from build123d import *

# Parameters (mm, degrees)
F0_W           = 85
F0_H           = 85
F0_W_2         = 80
F0_H_2         = 80
F1_DEPTH       = 5
F0_R           = 3.25
F2_DEPTH       = 2.5
F3_D           = 3
F3_CSINK_D     = 5.75
F3_CSINK_ANGLE = 90


with BuildPart() as f1:
    # F0 (on Top) → F1 (new body)
    with BuildSketch(Plane.XY):
        Rectangle(F0_W, F0_H)
        Rectangle(F0_W_2, F0_H_2, mode=Mode.SUBTRACT)
    extrude(amount=-F1_DEPTH)

    # F0 (on Top) → F2 (join)
    with BuildSketch(Plane.XY):
        Rectangle(F0_W_2, F0_H_2)
        with Locations((-35, -35)):
            Circle(F0_R, mode=Mode.SUBTRACT)
        with Locations((-25, -35)):
            Circle(F0_R, mode=Mode.SUBTRACT)
        with Locations((-35, -25)):
            Circle(F0_R, mode=Mode.SUBTRACT)
        with Locations((-15, -35)):
            Circle(F0_R, mode=Mode.SUBTRACT)
        with Locations((-5, -35)):
            Circle(F0_R, mode=Mode.SUBTRACT)
        with Locations((-15, -25)):
            Circle(F0_R, mode=Mode.SUBTRACT)
        with Locations((-5, -25)):
            Circle(F0_R, mode=Mode.SUBTRACT)
        with Locations((-35, -15)):
            Circle(F0_R, mode=Mode.SUBTRACT)
        with Locations((-25, -15)):
            Circle(F0_R, mode=Mode.SUBTRACT)
        with Locations((-35, -5)):
            Circle(F0_R, mode=Mode.SUBTRACT)
        with Locations((-25, -5)):
            Circle(F0_R, mode=Mode.SUBTRACT)
        with Locations((-15, -15)):
            Circle(F0_R, mode=Mode.SUBTRACT)
        with Locations((-5, -15)):
            Circle(F0_R, mode=Mode.SUBTRACT)
        with Locations((-15, -5)):
            Circle(F0_R, mode=Mode.SUBTRACT)
        with Locations((-5, -5)):
            Circle(F0_R, mode=Mode.SUBTRACT)
        with Locations((5, -35)):
            Circle(F0_R, mode=Mode.SUBTRACT)
        with Locations((15, -35)):
            Circle(F0_R, mode=Mode.SUBTRACT)
        with Locations((5, -25)):
            Circle(F0_R, mode=Mode.SUBTRACT)
        with Locations((15, -25)):
            Circle(F0_R, mode=Mode.SUBTRACT)
        with Locations((25, -35)):
            Circle(F0_R, mode=Mode.SUBTRACT)
        with Locations((35, -35)):
            Circle(F0_R, mode=Mode.SUBTRACT)
        with Locations((35, -25)):
            Circle(F0_R, mode=Mode.SUBTRACT)
        with Locations((5, -15)):
            Circle(F0_R, mode=Mode.SUBTRACT)
        with Locations((15, -15)):
            Circle(F0_R, mode=Mode.SUBTRACT)
        with Locations((5, -5)):
            Circle(F0_R, mode=Mode.SUBTRACT)
        with Locations((15, -5)):
            Circle(F0_R, mode=Mode.SUBTRACT)
        with Locations((25, -15)):
            Circle(F0_R, mode=Mode.SUBTRACT)
        with Locations((35, -15)):
            Circle(F0_R, mode=Mode.SUBTRACT)
        with Locations((25, -5)):
            Circle(F0_R, mode=Mode.SUBTRACT)
        with Locations((35, -5)):
            Circle(F0_R, mode=Mode.SUBTRACT)
        with Locations((-35, 5)):
            Circle(F0_R, mode=Mode.SUBTRACT)
        with Locations((-25, 5)):
            Circle(F0_R, mode=Mode.SUBTRACT)
        with Locations((-35, 15)):
            Circle(F0_R, mode=Mode.SUBTRACT)
        with Locations((-25, 15)):
            Circle(F0_R, mode=Mode.SUBTRACT)
        with Locations((-15, 5)):
            Circle(F0_R, mode=Mode.SUBTRACT)
        with Locations((-5, 5)):
            Circle(F0_R, mode=Mode.SUBTRACT)
        with Locations((-15, 15)):
            Circle(F0_R, mode=Mode.SUBTRACT)
        with Locations((-5, 15)):
            Circle(F0_R, mode=Mode.SUBTRACT)
        with Locations((-35, 25)):
            Circle(F0_R, mode=Mode.SUBTRACT)
        with Locations((-35, 35)):
            Circle(F0_R, mode=Mode.SUBTRACT)
        with Locations((-25, 35)):
            Circle(F0_R, mode=Mode.SUBTRACT)
        with Locations((-15, 25)):
            Circle(F0_R, mode=Mode.SUBTRACT)
        with Locations((-5, 25)):
            Circle(F0_R, mode=Mode.SUBTRACT)
        with Locations((-15, 35)):
            Circle(F0_R, mode=Mode.SUBTRACT)
        with Locations((-5, 35)):
            Circle(F0_R, mode=Mode.SUBTRACT)
        with Locations((5, 5)):
            Circle(F0_R, mode=Mode.SUBTRACT)
        with Locations((15, 5)):
            Circle(F0_R, mode=Mode.SUBTRACT)
        with Locations((5, 15)):
            Circle(F0_R, mode=Mode.SUBTRACT)
        with Locations((15, 15)):
            Circle(F0_R, mode=Mode.SUBTRACT)
        with Locations((25, 5)):
            Circle(F0_R, mode=Mode.SUBTRACT)
        with Locations((35, 5)):
            Circle(F0_R, mode=Mode.SUBTRACT)
        with Locations((25, 15)):
            Circle(F0_R, mode=Mode.SUBTRACT)
        with Locations((35, 15)):
            Circle(F0_R, mode=Mode.SUBTRACT)
        with Locations((5, 25)):
            Circle(F0_R, mode=Mode.SUBTRACT)
        with Locations((15, 25)):
            Circle(F0_R, mode=Mode.SUBTRACT)
        with Locations((5, 35)):
            Circle(F0_R, mode=Mode.SUBTRACT)
        with Locations((15, 35)):
            Circle(F0_R, mode=Mode.SUBTRACT)
        with Locations((35, 25)):
            Circle(F0_R, mode=Mode.SUBTRACT)
        with Locations((25, 35)):
            Circle(F0_R, mode=Mode.SUBTRACT)
        with Locations((35, 35)):
            Circle(F0_R, mode=Mode.SUBTRACT)
    extrude(amount=-F2_DEPTH)

    # F3 (through all)
    with Locations(Plane.XY):
        with Locations((-25, 25), (25, 25), (25, -25), (-25, -25)):
            CounterSinkHole(F3_D / 2, F3_CSINK_D / 2, counter_sink_angle=F3_CSINK_ANGLE)


solid = f1.part
Work out the finished part from the listing and answer in its coordinate system (mm). A direction names the side the tool comes from. Coordinates: 2 decimals unless noted, no trailing zeros. Order: outer loops, then holes, each group sorted by start corner. A loop starts at its lowest first (then second) coordinate and runs counter-clockwise, first axis right, second up. Notation, with made-up numbers: (31, 3) - (37, 3) arc R23 cw to (37, 29) - close; hole circle Ø6 at (55, 32.5). An arc over 180 degrees is marked (long way). Put each result on its own line as item: value. Start each with the question number.
1) Find the intervals of material crossed by line 1 (X direction, y = -16, z = -4.4); line 2 (Z direction, x = -16.5, y = 11), in increasing order. Write a range as from..to.
2) Find section A-A (y = 0). Give the vertices of the cut face in (x, z), plus the area to 3 significant figures.
3) For faces 3 (the cylindrical face through (-33.5, -37.883, -1.232)), 4 (the flat face through (-40, -1, -4)), determine the directions among +Z, -Z, +X, -X, +Y, -Y from which every point of the face is accessible in a straight line to the end or side of a thin tool.
4) For a pull along Y with two mould halves and no side action, classify faces 1 (the flat face through (-1, 1, 0)), 2 (the cylindrical face through (14.295, -38.173, -1.232)) as released by +Y, released by -Y, zero draft, split by the parting line, or undercut.
5) Flat-ended cylindrical pins translate along their axes: pin 1 (7.5 mm diameter, centred on x = -5, y = -35, fed in from -Z); pin 2 (4 mm diameter, centred on x = -35, y = -5, fed in from -Z). Find the tip coordinate at first contact, or state that the pin passes through.
6) Find section C-C (x = -5). State how many separate pieces and enclosed holes the cut face has, plus the area to 3 significant figures.
Results list:
1. line 1: x = -42.5..-40, 40..42.5
1. line 2: z = -2.5..0
2. outline: (-42.5, -5) - (-40, -5) - (-40, -2.5) - (40, -2.5) - (40, -5) - (42.5, -5) - (42.5, 0) - (-42.5, 0) - close
2. area: 225 mm^2
3. face 3: +Z, -Z
3. face 4: -Z
4. face 1: zero draft
4. face 2: undercut
5. pin 1: stops at z = -2.5
5. pin 2: passes through
6. separate pieces: 9
6. enclosed holes: 0
6. area: 95.0 mm^2
